Input: part model. Units: mm. Frame: model coordinates. A direction names the side the tool comes from. Coordinates: 2 decimals unless noted, no trailing zeros. Loops run counter-clockwise (first coordinate to the right, second up) from the corner with the lowest first, then second, coordinate; pieces in that order, holes last. Notation, with made-up numbers: (-25, 45) - (12, 45) arc R23 cw to (12, 80) - close; hole circle Ø8 at (48, -2). An arc over 180 degrees is marked (long way). Write item = value, one per line. Start each with the question number.
from build123d import *

# Parameters (mm, degrees)
F3_R     = 5.08
F4_R     = 12.573
F5_DEPTH = 5.08


with BuildPart() as f2:
    # F0 (on Front) → F2 section 0
    with BuildSketch(Plane.XZ, mode=Mode.PRIVATE) as f2_s0:
        Polygon((-44.901281, 0), (0, -44.901281), (44.901281, 0), (0, 44.901281), align=None)
    loft([f2_s0.sketch, Vertex(0, -20.32, 0)])

    # F3
    f3_edges = [f2.edges().sort_by_distance(p)[0] for p in [
        (-22.45064, 0, -22.45064),
        (22.45064, 0, -22.45064),
        (22.45064, 0, 22.45064),
        (-22.45064, 0, 22.45064),
    ]]
    fillet(f3_edges, radius=F3_R)

    # F4 (on face) → F5 (cut)
    with BuildSketch(Plane(origin=(0, 0, 0), x_dir=(-1, 0, 0), z_dir=(0, 1, 0))):
        Circle(F4_R)
    extrude(amount=-F5_DEPTH, mode=Mode.SUBTRACT)


solid = f2.part
Item 1: Ray query, line 1 (X direction, y = -2.25, z = 3); line 2 (Z direction, x = 1, y = -3.25); line 3 (Y direction, x = -8.5, z = -1). Return the intervals inside material, ascending.
Item 2: Cut plane A-A on y = -6.75. Return loops of the section in (x, z), plus the area to 3 significant figures.
Item 3: Pin query (flat end, axial travel): pin 1 (10 mm diameter, centred on x = -10, y = -14, fed in from -Z); pin 2 (6 mm diameter, centred on x = 13, z = -10, fed in from -Y); pin 3 (6 mm diameter, centred on y = -13.5, z = -7, fed in from +X); pin 4 (4 mm diameter, centred on x = -17.5, y = -16.5, fed in from -Z). Return the tip coordinate at first contact, or that it passes through.
Item 4: Access query for faces 1 (the flat face through (7.147, -13.698, -7.486)), 2 (the cylindrical face through (2.726, -2.504, -12.274)). Directions: +Z, -Z, +X, -X, +Y, -Y. A direction counts if a zero-diameter tool reaches every point of the face in a straight line with its end or side. Return the directions, or none.
Item 5: Cut plane B-B on y = -13.75. Return loops of the section in (x, z), plus the area to 3 significant figures.
Recorded:
q1.line_1 = -23.31 to -12.21, 12.21 to 23.31
q1.line_2 = -26.05 to -12.53, 12.53 to 26.05
q1.line_3 = -16.02 to -5.08
q2.outline = (-27.13, 0) - (0, -27.13) - (27.13, 0) - (0, 27.13) - close
q2.area = 1,470 mm²
q3.pin_1 = -16.09
q3.pin_2 = -11.83
q3.pin_3 = 15.35
q3.pin_4 = through
q4.face_1 = -Z, +X, -Y
q4.face_2 = +Y
q5.outline = (-14.52, 0) - (0, -14.52) - (14.52, 0) - (0, 14.52) - close
q5.area = 422 mm²
